Verification items for the finished model (mm, model axes). Face numbers are marked on the shaded views. A direction names the side the tool comes from. Round coordinates to 2 decimals unless told otherwise and drop trailing zeros. Loops run counter-clockwise (first coordinate to the right, second up) from the corner with the lowest first, then second, coordinate; pieces in that order, holes last. Notation, with made-up numbers: M -23.5,6 L -9.5,6 A27 ccw -9.5,42 Z; hole C 81,-7.5 d6. An arc over 180 degrees is marked long. Write item = value, one per line. Start each with the question number.
from build123d import *

# Parameters (mm, degrees)
F1_DEPTH = 63.5
F2_DEPTH = 25.4
F3_DEPTH = 15.875
F4_DEPTH = 25.4


with BuildPart() as f1:
    # F0 (on Front) → F1 (new body, symmetric)
    with BuildSketch(Plane.XZ):
        Polygon((-41.275, -9.525), (41.275, -9.525), (41.275, 9.525), (22.225, 9.525), (-41.275, 9.525), align=None)
    extrude(amount=F1_DEPTH, both=True)

    # F0 (on Front) → F2 (join, symmetric)
    with BuildSketch(Plane.XZ):
        with BuildLine():
            Line((22.225, 9.525), (41.275, 9.525))
            Line((41.275, 9.525), (41.275, 25.7178696878))
            ThreePointArc((41.275, 25.7178696878), (45.8998261561, 36.9182809964), (57.0796253206, 41.5927136998))
            Line((57.0796253206, 41.5927136998), (68.4412825856, 41.643080997))
            Line((68.4412825856, 41.643080997), (68.4412825856, 60.6932681845))
            Line((68.4412825856, 60.6932681845), (56.9951757054, 60.6425265141))
            ThreePointArc((56.9951757054, 60.6425265141), (32.3996175435, 50.3587745668), (22.225, 25.7178696878))
            Line((22.225, 25.7178696878), (22.225, 9.525))
        make_face()
    extrude(amount=F2_DEPTH, both=True)

    # F0 (on Front) → F3 (join)
    with BuildSketch(Plane.XZ):
        with BuildLine():
            add(Edge.make_bspline(
                [(-41.275, 9.525), (-37.726026519, 17.3571106564), (-29.2428259937, 36.0784016411), (18.3467226323, 68.3243904358), (51.9597658065, 67.2176628394), (68.4412825856, 66.675)],
                knots=[0, 0, 0, 0, 0.2682476731, 0.6411991562, 1, 1, 1, 1], degree=3))
            Line((-41.275, 9.525), (22.225, 9.525))
            Line((22.225, 9.525), (22.225, 25.7178696878))
            ThreePointArc((22.225, 25.7178696878), (32.3996175435, 50.3587745668), (56.9951757054, 60.6425265141))
            Line((56.9951757054, 60.6425265141), (68.4412825856, 60.6932681845))
            Line((68.4412825856, 60.6932681845), (68.4412825856, 66.675))
        make_face()
    extrude(amount=F3_DEPTH)

    # F0 (on Front) → F4 (join, symmetric)
    with BuildSketch(Plane.XZ):
        Polygon((93.7568329704, 60.8054944048), (68.4412825856, 60.6932681845), (68.4412825856, 41.643080997), (93.7676358867, 41.7553551076), (93.8239354557, 60.8052960923), align=None)
        Polygon((119.2412825856, 60.7301785005), (93.8239354557, 60.8052960923), (93.7676358867, 41.7553551076), (93.8412825856, 41.7556815904), (119.2412825856, 41.7556815904), align=None)
    extrude(amount=F4_DEPTH, both=True)

    # F0 (on Front) → F5 (revolve)
    with BuildSketch(Plane.XZ):
        Polygon((93.8412825856, 41.7556815904), (93.7676358867, 41.7553551076), (93.7568329704, 38.1), (119.2412825856, 38.1), (119.2412825856, 41.7556815904), align=None)
        Polygon((119.2412825856, 66.675), (93.8412825856, 66.675), (93.8239354557, 60.8052960923), (119.2412825856, 60.7301785005), align=None)
    revolve(axis=Axis((93.799057778, 0, 52.3875), (-0.0029553542, 0, -0.9999956329)))


solid = f1.part
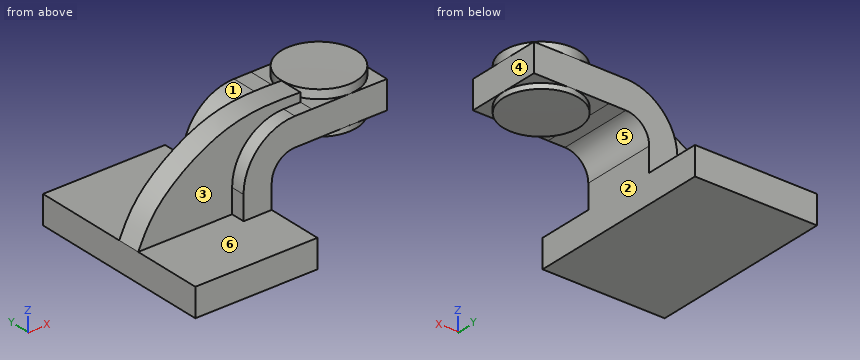
1. Thickness scan on line 1 (Z direction, x = 111, y = -12); line 2 (Y direction, x = -17, z = 14) (3 decimals); line 3 (Z direction, x = 33, y = 37) (3 decimals). Record the ranges inside material, lowest first.
2. Section check A-A, the plane z = 7.5. Enter the section's corners in (x, y) (3 decimals), and give its area (3 significant figures).
3. Tool access check on the marked faces 1, 2 and 3. Record the directions out of +Z, -Z, +X, -X, +Y, -Y that give a thin tool (end or side, any length) a straight path to the whole face; none if there is none.
4. Gauge pin test, flat ends, axial feed: P1, Ø24, axis at x = 8, y = -40, coming from the +Z side (3 decimals); P2, Ø7, axis at x = 111, y = 12.5, coming from the -Z side; P3, Ø10.5, axis at y = -22, z = 21, coming from the -X side (3 decimals). Record the tip position at first contact, or that the pin passes through.
5. Mould release check, pull along X, two halves, no side actions. Record for the marked faces 4, 5 and 6: pulls with the +X half, pulls with the -X half, needs draft (parallel to the pull), parting line crosses it, or undercut.
6. Section check B-B, the plane y = -31.5. Enter the section's corners in (x, z) (3 decimals).
Computed values:
q1.line_1 = 38.11 to 66.69
q1.line_2 = -15.875 to 0
q1.line_3 = -9.525 to 9.525
q2.outline = M -41.275,-63.5 L 41.275,-63.5 L 41.275,63.5 L -41.275,63.5 Z
q2.area = 10,500 mm2
q3.face_1 = +Z, -X, +Y
q3.face_2 = -Z, +X, +Y, -Y
q3.face_3 = +Z, -X, -Y
q4.P1 = 9.525
q4.P2 = 38.11
q4.P3 = 22.225
q5.face_4 = pulls with the +X half
q5.face_5 = undercut
q5.face_6 = needs draft
q6.outline = M -41.275,-9.525 L 41.275,-9.525 L 41.275,9.525 L -41.275,9.525 Z
